Part model, mm, in its own coordinate system. A direction names the side the tool comes from. Give positions to 0.01 mm unless a question says otherwise; leave off trailing zeros. Order: outer loops, then holes, each group sorted by start corner. A loop starts at its lowest first (then second) coordinate and runs counter-clockwise, first axis right, second up. Notation, with made-up numbers: (45, 53) -> (80, 53) arc R17 cw to (80, 76) -> close; hole circle Ø1 at (-34.5, 28). An arc over 180 degrees is marked (long way). Write item = value, one per line. Start each with the question number.
(1) Flat gauge pins, fed straight in: pin 1 (3 mm diameter, centred on x = 4, z = 218.5, fed in from +Y); pin 2 (0.6 mm diameter, centred on x = 14, y = 7, fed in from -Z); pin 3 (15 mm diameter, centred on y = 20.5, z = 230, fed in from -X); pin 4 (24 mm diameter, centred on y = 14, z = 129.5, fed in from -X). Where does each tip first touch, or does it go through?
(2) Probe line 1 along X through (y, z) = (17.5, 280); line 2 along Y through (x, z) = (-11, 417). List the from-to ranges inside material, lowest first. Write a range as from..to.
(3) Which spindle directions (+Z, -Z, +X, -X, +Y, -Y) get a long thin tool onto all of the face, cutting with end or side? Do faces 1 (the flat face through (0, 0, 0)), 2 (the flat face through (13, 19, 225)). Say none if no direction does.
(4) Saw through at A-A, the plane y = 21.5. State how many separate pieces and enclosed holes the cut face has, then the cut area to 3 significant figures.
(5) Saw through at B-B, the plane x = 1. List the corners of the cut face in (y, z).
from build123d import *

# Parameters (mm, degrees)
SKETCH1_W           = 30
SKETCH1_H           = 8
BOSS_EXTRUDE1_DEPTH = 50
SKETCH2_R           = 2
BOSS_EXTRUDE2_DEPTH = 2
LPATTERN1_COUNT     = 10
LPATTERN1_PITCH     = 50


with BuildPart() as part:
    # Sketch1 → Boss-Extrude1 (new body)
    with BuildSketch(Plane.XY):
        Rectangle(SKETCH1_W, SKETCH1_H)
    boss_extrude1 = extrude(amount=BOSS_EXTRUDE1_DEPTH)

    # Sketch2 → Boss-Extrude2 (add)
    with BuildSketch(Plane(origin=(15, 0, 0), x_dir=(0, 0, -1), z_dir=(1, 0, 0))):
        with BuildLine():
            Line((-40, 14), (-40, 4))
            Line((-40, 4), (-10, 4))
            Line((-10, 4), (-10, 14))
            add(Edge.make_bspline(
                [(-10, 14), (-22.549212794, 24.931170197), (-25, 41.661304797)],
                knots=[0, 0, 0, 1, 1, 1], degree=2))
            add(Edge.make_bspline(
                [(-40, 14), (-27.450787206, 24.931170197), (-25, 41.661304797)],
                knots=[0, 0, 0, 1, 1, 1], degree=2))
        make_face()
        with Locations((-25, 14)):
            Circle(SKETCH2_R, mode=Mode.SUBTRACT)
    boss_extrude2 = extrude(amount=-BOSS_EXTRUDE2_DEPTH)

    # LPattern1: Boss-Extrude1, Boss-Extrude2 ×10
    with Locations(*[(0, 0, i * LPATTERN1_PITCH) for i in range(1, LPATTERN1_COUNT)]):
        add(boss_extrude1)
        add(boss_extrude2)


solid = part.part
Results list:
q1.pin_1 = 4
q1.pin_2 = 10
q1.pin_3 = 13
q1.pin_4 = -15
q2.line_1 = 13..15
q2.line_2 = -4..4
q3.face_1 = -Z, +X, -X, +Y, -Y
q3.face_2 = +Z, -Z, -X, +Y
q4.separate_pieces = 10
q4.enclosed_holes = 0
q4.area = 323 mm^2
q5.outline = (-4, 0) -> (4, 0) -> (4, 500) -> (-4, 500) -> close
